```python
from build123d import *

# Parameters (mm, degrees)
PAD_DEPTH    = 3
SKETCH001_R  = 16
PAD001_DEPTH = 20
SKETCH002_R  = 14
POCKET_DEPTH = 18
SKETCH003_R  = 3.8
PAD002_DEPTH = 10


with BuildPart() as part:
    # Sketch → Pad (new body)
    with BuildSketch(Plane.XY):
        with BuildLine():
            Line((-125.969839, 5.652203), (-105.955548, 12.728901))
            ThreePointArc((-87.587906, 15.880533), (-96.90594, 15.08691), (-105.955548, 12.728901))
            Line((-87.587906, 15.880533), (-56.304531, 15.880533))
            Line((-56.304531, 15.880533), (67.96893, 15.880533))
            ThreePointArc((67.96893, 15.880533), (79.23833, 19.445245), (86.407644, 28.842452))
            Line((86.407644, 28.842452), (101.576416, 71.003891))
            Line((101.576416, 71.003891), (125, 71.003891))
            Line((125, 71.003891), (125, 0))
            Line((125, 0), (-125, 0))
            ThreePointArc((-125.969839, 5.652203), (-127.867402, 2.4173), (-125, 0))
        make_face()
    extrude(amount=PAD_DEPTH)

    # Sketch001 (on Face9 of Pad) → Pad001 (join)
    with BuildSketch(Plane.XZ):
        Circle(SKETCH001_R)
    extrude(amount=PAD001_DEPTH)

    # Sketch002 (on Face17 of Pad001) → Pocket (cut)
    with BuildSketch(Plane.XZ.offset(20)):
        Circle(SKETCH002_R)
    extrude(amount=-POCKET_DEPTH, mode=Mode.SUBTRACT)

    # Sketch003 (on Face19 of Pocket) → Pad002 (join)
    with BuildSketch(Plane.XZ.offset(2)):
        Circle(SKETCH003_R)
    extrude(amount=PAD002_DEPTH)


solid = part.part
```
Check sheet for the modelled part. Datum: model origin and axes. Units: mm. A direction names the side the tool comes from. Coordinates: 2 decimals unless noted, no trailing zeros. Write each loop counter-clockwise with the first axis right and the second up, starting at its lowest first coordinate (ties: lowest second). Pieces come first, ordered by that corner, then holes. Notation, with made-up numbers: M 49.25,68 L 59.25,68 A29 cw 59.25,89 Z; hole C 68,-23 d10. An arc over 180 degrees is marked long. Write item = value, one per line. Start each with the question number.
1. Sectioned sample at A-A (x = 0). Record the cut outline in (y, z), then the cut area to 3 significant figures.
2. Sectioned sample at B-B (y = -5). Record the cut outline in (x, z), then the cut area to 3 significant figures.
3. Tool access check on faces 4 (the flat face through (0, 0, 8)), 5 (the flat face through (-116.1, 9.14, 1.48)), 6 (the cylindrical face through (-3.796, -6.93, 0.167)). Record the directions out of +Z, -Z, +X, -X, +Y, -Y that give a thin tool (end or side, any length) a straight path to the whole face; none if there is none.
4. Thickness scan on probe 1 along Z at (x, y) = (0, -13); probe 2 along X at (y, z) = (-15, 5). Record the ranges inside material, lowest first.
5. Mould release check, pull along Z, two halves, no side actions. Record for faces 1 (the cylindrical face through (-3.47, -9.86, -15.62)), 2 (the flat face through (0, 0, -6)), 3 (the flat face through (0, -12, 0)): pulls with the +Z half, pulls with the -Z half, needs draft (parallel to the pull), parting line crosses it, or undercut.
6. Sectioned sample at C-C (z = 7.5). Record the cut outline in (x, y).
7. Sectioned sample at D-D (y = 9.5). Record the cut outline in (x, z).
8. Go/stop test with flat-tipped pins: pin 1 (1.5 mm diameter, centred on x = -13.5, y = 2, fed in from -Z); pin 2 (4 mm diameter, centred on x = 0, z = -1, fed in from -Y); pin 3 (12 mm diameter, centred on x = 14.5, z = 11, fed in from -Y); pin 4 (3.5 mm diameter, centred on x = -88, z = 2, fed in from -Y). Record where each tip stops, or that it passes through.
The answers:
q1.outline = M -20,-16 L 0,-16 L 0,0 L 15.88,0 L 15.88,3 L 0,3 L 0,16 L -20,16 L -20,14 L -2,14 L -2,3.8 L -12,3.8 L -12,-3.8 L -2,-3.8 L -2,-14 L -20,-14 Z
q1.area = 260 mm²
q2.outline = C 0,0 d32; C 0,0 d7.6; hole C 0,0 d28
q2.area = 234 mm²
q3.face_4 = +Z, +X, -X, +Y
q3.face_5 = +Z, -Z, -X, +Y
q3.face_6 = -Y
q4.probe_1 = -16 to -14, 14 to 16
q4.probe_2 = -15.2 to -13.08, 13.08 to 15.2
q5.face_1 = parting line crosses it
q5.face_2 = needs draft
q5.face_3 = undercut
q6.outline = M -14.13,-20 L -11.82,-20 L -11.82,-2 L 11.82,-2 L 11.82,-20 L 14.13,-20 L 14.13,0 L -14.13,0 Z
q7.outline = M -115.09,0 L 125,0 L 125,3 L -115.09,3 Z
q8.pin_1 = 0
q8.pin_2 = -12
q8.pin_3 = -20
q8.pin_4 = 0
